from build123d import *

# Parameters (mm, degrees)
F1_DEPTH = 10
F2_SIZE2 = 0.5
F2_SIZE  = 2
F4_DEPTH = 3
F5_R     = 1


with BuildPart() as f1:
    # F0 (on Top) → F1 (new body)
    with BuildSketch(Plane.XY):
        with BuildLine():
            Line((3.75, 2.75), (-3.75, 2.75))
            ThreePointArc((-3.75, 2.75), (-2.4130258043, 2.4031229681), (-1.4133357109, 1.45))
            Line((-1.4133357109, 1.45), (1.4133357109, 1.45))
            ThreePointArc((1.4133357109, 1.45), (2.4130258043, 2.4031229681), (3.75, 2.75))
        make_face()
        with BuildLine():
            ThreePointArc((-1.4133357109, 1.45), (-2.4130258043, 2.4031229681), (-3.75, 2.75))
            ThreePointArc((-3.75, 2.75), (-6.5, 0), (-3.75, -2.75))
            ThreePointArc((-3.75, -2.75), (-2.4130258043, -2.4031229681), (-1.4133357109, -1.45))
            Line((-1.4133357109, -1.45), (-4.1, -1.45))
            Line((-4.1, -1.45), (-4.1, 1.45))
            Line((-4.1, 1.45), (-1.4133357109, 1.45))
        make_face()
        with BuildLine():
            ThreePointArc((6.5, 0), (5.6945436483, 1.9445436483), (3.75, 2.75))
            ThreePointArc((3.75, 2.75), (2.4130258043, 2.4031229681), (1.4133357109, 1.45))
            Line((1.4133357109, 1.45), (4.1, 1.45))
            Line((4.1, 1.45), (4.1, -1.45))
            Line((4.1, -1.45), (1.4133357109, -1.45))
            ThreePointArc((1.4133357109, -1.45), (2.4130258043, -2.4031229681), (3.75, -2.75))
            ThreePointArc((3.75, -2.75), (5.6945436483, -1.9445436483), (6.5, 0))
        make_face()
        with BuildLine():
            ThreePointArc((-1.4133357109, -1.45), (-2.4130258043, -2.4031229681), (-3.75, -2.75))
            Line((-3.75, -2.75), (3.75, -2.75))
            ThreePointArc((3.75, -2.75), (2.4130258043, -2.4031229681), (1.4133357109, -1.45))
            Line((1.4133357109, -1.45), (-1.4133357109, -1.45))
        make_face()
    extrude(amount=F1_DEPTH)

    # F2
    f2_edges = [f1.edges().sort_by_distance(p)[0] for p in [
        (0, -2.75, 10),
    ]]
    f2_side = f1.faces().sort_by_distance((0, -2.75, 5))[0]
    chamfer(f2_edges, length=F2_SIZE, length2=F2_SIZE2, reference=f2_side)

    # F3 (on face) → F4 (join)
    with BuildSketch(Plane(origin=(0, 0, 0), x_dir=(1, 0, 0), z_dir=(0, 0, -1))):
        with BuildLine():
            ThreePointArc((3.75, -4.75), (8.5, 0), (3.75, 4.75))
            Line((3.75, 4.75), (-3.75, 4.75))
            ThreePointArc((-3.75, 4.75), (-8.5, 0), (-3.75, -4.75))
            Line((-3.75, -4.75), (3.75, -4.75))
        make_face()
        with BuildLine():
            Line((3.75, -2.75), (-3.75, -2.75))
            ThreePointArc((-3.75, -2.75), (-6.5, 0), (-3.75, 2.75))
            Line((-3.75, 2.75), (3.75, 2.75))
            ThreePointArc((3.75, 2.75), (6.5, 0), (3.75, -2.75))
        make_face(mode=Mode.SUBTRACT)
    extrude(amount=-F4_DEPTH)

    # F5
    f5_edges = [f1.edges().sort_by_distance(p)[0] for p in [
        (0, -4.75, 0),
        (8.5, 0, 0),
        (0, 4.75, 0),
    ]]
    fillet(f5_edges, radius=F5_R)


solid = f1.part
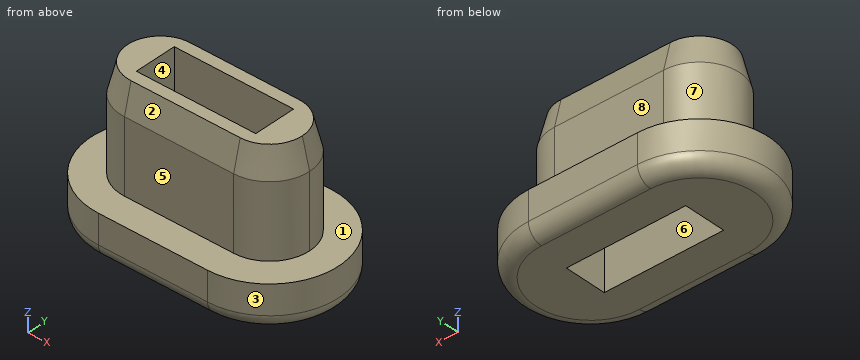
Can you work these out from the model? Positions are in its coordinate system, mm. Face numbers are marked on the shaded views. A direction names the side the tool comes from. Give positions to 0.01 mm unless a question says otherwise; leave off trailing zeros. Loops run counter-clockwise (first coordinate to the right, second up) from the corner with the lowest first, then second, coordinate; pieces in that order, holes last. Notation, with made-up numbers: (66, 6) - (108, 6) arc R18 cw to (108, 33) - close; hole circle Ø2 at (-12, 31.5). An arc over 180 degrees is marked (long way). Answer as a JSON object with one key per item and string values.
Q1. If we mould it in two halves opening along Y, with no side actions, what happens to the marked faces 1, 2, 3 and 4? For each: pulls with the +Y half, pulls with the -Y half, needs draft (parallel to the pull), parting line crosses it, or undercut.
Geometry says:
{"face 1": "needs draft", "face 2": "pulls with the -Y half", "face 3": "parting line crosses it", "face 4": "undercut"}
Q2. If I drill on L1, parallel to Y at x = 1.75, z = 2.5; L2, parallel to X at y = 0, z = 5; L3, parallel to X at y = 0, z = 1, over which ranges is the centre line in solid material (lowest first)?
Geometry says:
{"L1": "-4.75 to -1.45, 1.45 to 4.75", "L2": "-6.5 to -4.1, 4.1 to 6.5", "L3": "-8.5 to -4.1, 4.1 to 8.5"}
Q3. Imagine slicing it at B-B on z = 6.75. Write out the boundary of the cut face in (x, y).
Geometry says:
{"outline": "(-3.75, -2.75) - (3.75, -2.75) arc R2.75 ccw to (3.75, 2.75) - (-3.75, 2.75) arc R2.75 ccw to start; hole (-4.1, -1.45) - (4.1, -1.45) - (4.1, 1.45) - (-4.1, 1.45) - close"}
Q4. Will these pins go through, and if not, where does the flat tip stop? P1, Ø5, axis at x = 2.5, z = 6, coming from the +Y side; P2, Ø1.5, axis at x = 0, z = 6, coming from the -Y side; P3, Ø2.5, axis at y = -0.5, z = 4.5, coming from the +X side.
Geometry says:
{"P1": "y = 2.75", "P2": "y = -2.75", "P3": "x = 6.5"}
Q5. Which directions (+Z, -Z, +X, -X, +Y, -Y) give clear straight access to the entire face, cutting with the end or side of a thin tool? Please do the marked faces 5, 6, 7 and 8.
Geometry says:
{"face 5": "+Z, +X, -X, -Y", "face 6": "+Z, -Z", "face 7": "+Z, -X", "face 8": "+Z, +X, -X, +Y"}
Q6. Imagine slicing it at A-A on x = 0.5. Write out the boundary of the cut face in (y, z), plus the area to 3 significant figures.
Geometry says:
{"outline": "(-4.75, 1) arc R1 ccw to (-3.75, 0) - (-1.45, 0) - (-1.45, 10) - (-2.25, 10) - (-2.75, 8) - (-2.75, 3) - (-4.75, 3) - close; (1.45, 0) - (3.75, 0) arc R1 ccw to (4.75, 1) - (4.75, 3) - (2.75, 3) - (2.75, 8) - (2.25, 10) - (1.45, 10) - close", "area": "36.6 mm²"}
